Could you check a few things on this model? Use its own coordinates, in mm. A direction names the side the tool comes from. Give positions to 0.01 mm unless a question says otherwise; leave off trailing zeros. Order: outer loops, then holes, each group sorted by start corner. A loop starts at its lowest first (then second) coordinate and runs counter-clockwise, first axis right, second up. Notation, with made-up numbers: M 6.5,56.25 L 61.5,56.25 A21 cw 61.5,75.25 Z; hole C 15.25,55 d5. An arc over 180 degrees is marked long. Use a Markdown table: item, result. Add a question column.
```python
from build123d import *

# Parameters (mm, degrees)
SKETCH1_R                  = 14
SKETCH1_R_2                = 3
BOSS_EXTRUDE1_DEPTH        = 3
M1_6_CLEARANCE_HOLE2_D     = 1.8
M1_6_CLEARANCE_HOLE2_DEPTH = 11.5
CIRPATTERN1_COUNT          = 12
TROU_TARAUD_M1_61_D        = 1.25
CHAMFER2_SIZE              = 11.586303909
ESQUISSE1_R                = 21
ENL_V_MAT_EXTRU_1_DEPTH    = 10
ESQUISSE3_R                = 0.625
ENL_V_MAT_EXTRU_2_DEPTH    = 69.11418111
ESQUISSE5_W                = 15
ESQUISSE5_H                = 1.5
ENL_V_MAT_EXTRU_3_DEPTH    = 1.6
ENL_V_START                = -10
ENL_V_MAT_EXTRU_4_DEPTH    = 10
CONG_1_R                   = 2
BOSS_EXTRU_1_START         = -3
BOSS_EXTRU_1_DEPTH         = 3
CONG_2_R                   = 5
CONG_3_R                   = 0.5


with BuildPart() as part:
    # Sketch1 → Boss-Extrude1 (new body)
    with BuildSketch(Plane.XY):
        with BuildLine():
            Line((18.027756377, 6), (62.113532193, 4.998710878))
            ThreePointArc((62.113532193, 4.998710878), (67, 0), (62.113532193, -4.998710878))
            Line((62.113532193, -4.998710878), (18.027756377, -6))
            ThreePointArc((18.027756377, -6), (-19, 0), (18.027756377, 6))
        make_face()
        Circle(SKETCH1_R, mode=Mode.SUBTRACT)
        with Locations((46.5, 0)):
            Circle(SKETCH1_R_2, mode=Mode.SUBTRACT)
        with Locations((62, 0)):
            Circle(SKETCH1_R_2, mode=Mode.SUBTRACT)
    extrude(amount=BOSS_EXTRUDE1_DEPTH)

    # M1.6 Clearance Hole2
    with Locations(Plane.XY.offset(3)):
        with Locations((0, 16.5)):
            m1_6_clearance_hole2 = Hole(M1_6_CLEARANCE_HOLE2_D / 2, depth=M1_6_CLEARANCE_HOLE2_DEPTH)

    # CirPattern1: M1.6 Clearance Hole2 ×12 about axis
    cirpattern1_axis = Axis((0, 0, 0), (0, 0, 1))
    for i in range(1, CIRPATTERN1_COUNT):
        add(m1_6_clearance_hole2.rotate(cirpattern1_axis, i * 360 / CIRPATTERN1_COUNT), mode=Mode.SUBTRACT)

    # Trou taraudé M1.61 (through all)
    with Locations(Plane.XY.offset(3)):
        with Locations((38.75, 2.5), (54.25, -2.5), (38.75, -2.5), (54.25, 2.5)):
            Hole(TROU_TARAUD_M1_61_D / 2)

    # Chamfer2
    # the kernel refuses this chamfer: 11.586303909, 7 mm, written as the material it adds along each edge
    with BuildSketch(Plane(origin=(18.027756377, -6, 0), x_dir=(-0.5533672821308996, -0.8329373632315106, 0), z_dir=(0, 0, 1))) as chamfer2_piece_1:
        with BuildLine():
            Line((9.95669274, 0), (-CHAMFER2_SIZE * 0.572137651701, CHAMFER2_SIZE * 0.820157611387))
            Line((-CHAMFER2_SIZE * 0.572137651701, CHAMFER2_SIZE * 0.820157611387), (0, 0))
            ThreePointArc((0, 0), (5.187993151, 0.662647785), (9.95669274, 0))
        make_face()
    extrude(amount=3)
    with BuildSketch(Plane(origin=(18.027756377, 6, 0), x_dir=(0.9997421755844867, -0.02270643868151269, 0), z_dir=(0, 0, 1))) as chamfer2_piece_2:
        with BuildLine():
            Line((CHAMFER2_SIZE, 0), (-5.696598803, 8.166057335))
            ThreePointArc((-5.696598803, 8.166057335), (-2.424770594, 4.634097818), (0, 0))
            Line((0, 0), (CHAMFER2_SIZE, 0))
        make_face()
    extrude(amount=3)

    # Esquisse1 → Enlèv. mat.-Extru.1 (cut)
    with BuildSketch(Plane(origin=(0, 0, 0), x_dir=(-1, 0, 0), z_dir=(0, 0, -1))):
        Circle(ESQUISSE1_R)
    extrude(amount=-ENL_V_MAT_EXTRU_1_DEPTH, mode=Mode.SUBTRACT)

    # Esquisse3 → Enlèv. mat.-Extru.2 (cut, through all)
    with BuildSketch(Plane(origin=(0, 0, 0), x_dir=(-1, 0, 0), z_dir=(0, 0, -1))):
        with Locations((-25.251835753, 3.548914074)):
            Circle(ESQUISSE3_R)
        with Locations((-25.251835753, -3.548914074)):
            Circle(ESQUISSE3_R)
    extrude(amount=-ENL_V_MAT_EXTRU_2_DEPTH, mode=Mode.SUBTRACT)

    # Esquisse5 → Enlèv. mat.-Extru.3 (cut)
    with BuildSketch(Plane.XY.offset(3)):
        with Locations((58.5, 0)):
            Rectangle(ESQUISSE5_W, ESQUISSE5_H)
    extrude(amount=-ENL_V_MAT_EXTRU_3_DEPTH, mode=Mode.SUBTRACT)

    # Esquisse9 → Enlèv. mat.-Extru.4 (cut)
    with BuildSketch(Plane.XY.offset(3).offset(ENL_V_START)):
        with BuildLine():
            Line((22.5, 9.296560112), (19.409678401, 8.016506993))
            ThreePointArc((19.409678401, 8.016506993), (18.459529223, 10.012281501), (17.304864396, 11.897128572))
            Line((17.304864396, 11.897128572), (22.5, 9.296560112))
        make_face()
    extrude(amount=ENL_V_MAT_EXTRU_4_DEPTH, mode=Mode.SUBTRACT)

    # Congé1
    cong_1_edges = [part.edges().sort_by_distance(p)[0] for p in [
        (19.409678401, 8.016506993, 1.5),
    ]]
    fillet(cong_1_edges, radius=CONG_1_R)

    # Esquisse10 → Boss.-Extru.1 (add)
    with BuildSketch(Plane.XY.offset(3).offset(BOSS_EXTRU_1_START)):
        Polygon((31, 5.705370583), (23.569752194, 9.739665979), (22.5, 9.296560112), (29.611073054, 5.736916301), align=None)
        with BuildLine():
            Line((31, -5.705370583), (29.611073054, -5.736916301))
            Line((29.611073054, -5.736916301), (17.304864396, -11.897128572))
            ThreePointArc((17.304864396, -11.897128572), (16.480984157, -13.014498116), (15.585077408, -14.074990664))
            Line((15.585077408, -14.074990664), (31, -5.705370583))
        make_face()
    extrude(amount=BOSS_EXTRU_1_DEPTH)

    # Congé2
    cong_2_edges = [part.edges().sort_by_distance(p)[0] for p in [
        (31, 5.705370583, 1.5),
        (31, -5.705370583, 1.5),
    ]]
    fillet(cong_2_edges, radius=CONG_2_R)

    # Congé3
    cong_3_edges = [part.edges().sort_by_distance(p)[0] for p in [
        (15.585077408, -14.074990664, 1.5),
    ]]
    fillet(cong_3_edges, radius=CONG_3_R)


solid = part.part
```
1) Please list where these lines run through material, in increasing order: line 1 (X direction, y = -1.5, z = 2.8); line 2 (X direction, y = 1.75, z = 2.6); line 3 (Y direction, x = 54.25, z = 0.8) (3 decimals). Write a range as from..to.
2) For faces 1 (the face through (42, -1, 3)), 2 (the face through (55, 0, 1.4)), which set-ups out of +Z, -Z, +X, -X, +Y, -Y let a thin tool reach every point of the face, with its end or its side?
3) For pin 1 (1.6 mm diameter, centred on x = 38.75, y = 2.5, fed in from +Z); pin 2 (0.8 mm diameter, centred on y = -0.5, z = 2, fed in from -X); pin 3 (0.5 mm diameter, centred on x = 56, z = 2.5, fed in from +Y); pin 4 (0.5 mm diameter, centred on x = 55.5, z = 2.5, fed in from -Y), each with a flat end and sliding along its axis, tell me the tip position at first contact or that it passes through.
4) Suppose I cut it at B-B on x = 54.25. Please give me the cut outline in (y, z) (3 decimals).
5) We'd pull the mould along Y, two halves only. Please class faces 3 (the face through (31.05, -5.84, 1.52)), 4 (the face through (31.02, 5.85, 1.52)), 5 (the face through (53.673, -2.739, 1.479)): pulls with the +Y half, pulls with the -Y half, needs draft (parallel to the pull), parting line crosses it, or undercut.
6) Suppose I cut it at A-A on x = 63. Please give me the cut outline in (y, z).
7) Suppose I cut it at D-D on y = 6.75. Please give me the cut outline in (x, z).
8) Suppose I cut it at C-C on z = 1.85. Count the separate pieces of the cut face and the enclosed holes in it, and give its area (3 significant figures).
Values found:
| question | item | result |
|---|---|---|
| 1 | line 1 | x = 20.95..43.9, 49.1..59.4, 64.6..66.77 |
| 1 | line 2 | x = 20.93..44.06, 48.94..59.56, 64.44..66.68 |
| 1 | line 3 | y = -5.177..-3.125, -1.875..1.875, 3.125..5.177 |
| 2 | face 1 | +Z, +X, -X, +Y, -Y |
| 2 | face 2 | +Z |
| 3 | pin 1 | stops at z = 3 |
| 3 | pin 2 | stops at x = 20.98 |
| 3 | pin 3 | stops at y = 5.14 |
| 3 | pin 4 | stops at y = -5.15 |
| 4 | outline | M -5.177,0 L -3.125,0 L -3.125,3 L -5.177,3 Z; M -1.875,0 L 1.875,0 L 1.875,3 L 0.75,3 L 0.75,1.4 L -0.75,1.4 L -0.75,3 L -1.875,3 Z; M 3.125,0 L 5.177,0 L 5.177,3 L 3.125,3 Z |
| 5 | face 3 | pulls with the -Y half |
| 5 | face 4 | pulls with the +Y half |
| 5 | face 5 | undercut |
| 6 | outline | M -4.9,0 L -2.83,0 L -2.83,3 L -4.9,3 Z; M 2.83,0 L 4.9,0 L 4.9,3 L 2.83,3 Z |
| 7 | outline | M 19.95,0 L 29.08,0 L 29.08,3 L 19.95,3 Z |
| 8 | separate pieces | 1 |
| 8 | enclosed holes | 8 |
| 8 | area | 478 mm^2 |
